from build123d import *

# Parameters (mm, degrees)
SKETCH010_W     = 80
SKETCH010_H     = 110
PAD010_DEPTH    = 3
SKETCH034_R     = 2.000703
SKETCH034_R_2   = 1.961844
SKETCH034_R_3   = 2.000693
SKETCH034_R_4   = 2.053285
POCKET013_DEPTH = 5
SKETCH009_R     = 1.482535
SKETCH009_R_2   = 1.48253
SKETCH009_R_3   = 1.51367
SKETCH009_R_4   = 1.468475
POCKET014_DEPTH = 5


with BuildPart() as part:
    # Sketch010 → Pad010 (new body)
    with BuildSketch(Plane(origin=(100, 0, 403), x_dir=(1, 0, 0), z_dir=(0, 0, -1))):
        with Locations((68.06718, 204.993062)):
            Rectangle(SKETCH010_W, SKETCH010_H)
    extrude(amount=PAD010_DEPTH)

    # Sketch034 → Pocket013 (cut)
    with BuildSketch(Plane(origin=(100, 0, 400), x_dir=(1, 0, 0), z_dir=(0, 0, -1))):
        with Locations((32.289825, 250)):
            Circle(SKETCH034_R)
        with Locations((102.48175, 250)):
            Circle(SKETCH034_R_2)
        with Locations((34.151398, 160)):
            Circle(SKETCH034_R_3)
        with Locations((104.124298, 160)):
            Circle(SKETCH034_R_4)
    extrude(amount=-POCKET013_DEPTH, mode=Mode.SUBTRACT)

    # Sketch009 → Pocket014 (cut)
    with BuildSketch(Plane(origin=(100, 0, 400), x_dir=(1, 0, 0), z_dir=(0, 0, -1))):
        with Locations((91.958268, 230.158066)):
            Circle(SKETCH009_R)
        with Locations((91.375338, 181.883286)):
            Circle(SKETCH009_R_2)
        with Locations((40.37064, 196.380576)):
            Circle(SKETCH009_R_3)
        with Locations((40, 224.378723)):
            Circle(SKETCH009_R_4)
    extrude(amount=-POCKET014_DEPTH, mode=Mode.SUBTRACT)


solid = part.part
Geometry: final body of the model. Coordinates: model frame, mm. Give positions to 0.01 mm unless a question says otherwise; leave off trailing zeros. Loops run counter-clockwise (first coordinate to the right, second up) from the corner with the lowest first, then second, coordinate; pieces in that order, holes last. Notation, with made-up numbers: M 18,-1 L 36,-1 A20 cw 36,30 Z; hole C -4.5,34.25 d1. An arc over 180 degrees is marked long. Put each result on its own line as item: value. Start each with the question number.
1) Cut plane A-A (y = -250). Output: boundary loops of the cut face in (x, z), then the cut area to 3 significant figures.
2) Contact query for a flat-ended pin moving along its axis: pin 1 (3.5 mm diameter, centred on x = 134.15, y = -160, fed in from +Z). Output: stop coordinate, or through.
3) Cut plane B-B (y = -160). Output: boundary loops of the cut face in (x, z).
4) Ray query, line 1 along X through (y, z) = (-160, 401.15); line 2 along X through (y, z) = (-250, 401.45); line 3 along Y through (x, z) = (140, 401.05). Return the intervals inside material, ascending.
5) Pull-direction query (Y, two-part tool) for faces 1 (the flat face through (128.067, -204, 402)), 2 (the cylindrical face through (191.64, -228.71, 401.48)), 3 (the flat face through (168, -259.993, 402)), 4 (the cylindrical face through (192.8, -182.3, 401.5)); classes: pulls with the +Y half, pulls with the -Y half, needs draft (parallel to the pull), parting line crosses it, or undercut.
Verdict:
1. outline: M 128.07,400 L 130.29,400 L 130.29,403 L 128.07,403 Z; M 134.29,400 L 200.52,400 L 200.52,403 L 134.29,403 Z; M 204.44,400 L 208.07,400 L 208.07,403 L 204.44,403 Z
1. area: 216 mm2
2. pin 1: through
3. outline: M 128.07,400 L 132.15,400 L 132.15,403 L 128.07,403 Z; M 136.15,400 L 202.07,400 L 202.07,403 L 136.15,403 Z; M 206.18,400 L 208.07,400 L 208.07,403 L 206.18,403 Z
4. line 1: 128.07 to 132.15, 136.15 to 202.07, 206.18 to 208.07
4. line 2: 128.07 to 130.29, 134.29 to 200.52, 204.44 to 208.07
4. line 3: -259.99 to -225.85, -222.91 to -197.85, -194.91 to -149.99
5. face 1: needs draft
5. face 2: undercut
5. face 3: pulls with the -Y half
5. face 4: undercut
